Geometry: final body of the model. Coordinates: model frame, mm. Give positions to 0.01 mm unless a question says otherwise; leave off trailing zeros. Write each loop counter-clockwise with the first axis right and the second up, starting at its lowest first coordinate (ties: lowest second). Pieces come first, ordered by that corner, then holes.
Autodesk Inventor part; units mm, degrees
ref_plane "YZ Plane" through (0, 0, 0) normal (1, 0, 0) x (0, 1, 0)
ref_plane "XZ Plane" through (0, 0, 0) normal (0, 1, 0) x (-1, 0, 0)
ref_plane "XY Plane" through (0, 0, 0) normal (0, 0, 1) x (1, 0, 0)
sketch "Sketch1" plane through (0, 0, 0) normal (0, 1, 0) x (-1, 0, 0)
  line L0 (600, 0) -> (600, -21)
  arc A0 (523.9158, -145.5583) -> (600, -21) centre (460, -21) ccw
  arc A1 (17.5, -272) -> (523.9158, -145.5583) centre (0, 875.442) ccw
  line L1 (0, 272) -> (0, -272)
  arc A2 (17.5, -265.9993) -> (521.1766, -140.2201) centre (0, 875.442) ccw
  arc A3 (521.1766, -140.2201) -> (594, -21) centre (460, -21) ccw
  line L2 (594, -21) -> (594, 0)
  line L3 (594, 0) -> (600, 0)
  line L4 (0, -272) -> (17.5, -272)
  line L5 (0, -265.9993) -> (17.5, -265.9993)
  line L6 (17.5, -272) -> (17.5, -265.9993)
  point P0 (0, 0)
  point P1 (0, 0)
  point P2 (0, -163.7009)
  point P3 (0, -169.7009)
  dimension "d0" = 140
  dimension "d1" = 21
  dimension "d3" = 1147.5754
  dimension "d6" = 6
  dimension "d13" = 35
  dimension "d14" = 1200
  dimension "d15" = 272
revolve "Revolution1" add sketch "Sketch1" angle 360 about axis through (0, 0, 272) along (0, 0, -1) contours L0 A0 A1 L6 A2 A3 L2 L3
equation "\"d0\" = tech_dishhead_small_rad"
equation "\"d1\" = tech_dishhead_edge_hight"
equation "\"d13\" = tech_dishhead_bottom_hole"
equation "\"d14\" = MAIN_filter_diam"
properties part number "TZS 1208 dished head" material "Steel"
Item 1: Pin query (flat end, axial travel): pin 1 Ø5 at (x, z) = (83, -28) entering from -Y; pin 2 Ø2 at (x, y) = (253, -200.5) entering from +Z; pin 3 Ø4 at (x, y) = (-46.5, -390.5) entering from -Z. Return the tip coordinate at first contact, or that it passes through.
Found:
pin 1: stops at y = -594.42
pin 2: stops at z = -219.24
pin 3: stops at z = -203.37
Item 2: Pull-direction query (X, two-part tool) for faces 1 (the face through (581, 136, 0)), 2 (the face through (13.887, 10.648, -268.958)), 3 (the face through (78.108, 594.894, -10.647)); classes: +X half, -X half, draft (parallel to the pull), parting line (faces both ways), or undercut.
Found:
face 1: draft
face 2: undercut
face 3: parting line
Item 3: Line query: L1, parallel to Y at x = 0, z = -7.75; L2, parallel to X at y = 332, z = -91.5; L3, parallel to Y at x = 241.5, z = -23. Output: solid intervals per line, ascending.
Found:
L1: y = -600 to -594, 594 to 600
L2: x = -476.74 to -468.19, 468.19 to 476.74
L3: y = -549.24 to -542.67, 542.67 to 549.24
Item 4: Section A-A, the plane z = -54.5. Return the cut outline in (x, y), plus the area to 3 significant figures.
Found:
outline: circle Ø1191.87 at (0, 0); hole circle Ø1179.49 at (0, 0)
area: 23,000 mm2
